Read the model definition and answer for the solid it produces. Units are mm, in the model's axes. Face numbers are marked on the shaded views. A direction names the side the tool comes from. Round coordinates to 2 decimals unless told otherwise and drop trailing zeros. Write each loop counter-clockwise with the first axis right and the second up, starting at its lowest first coordinate (ties: lowest second). Pieces come first, ordered by that corner, then holes.
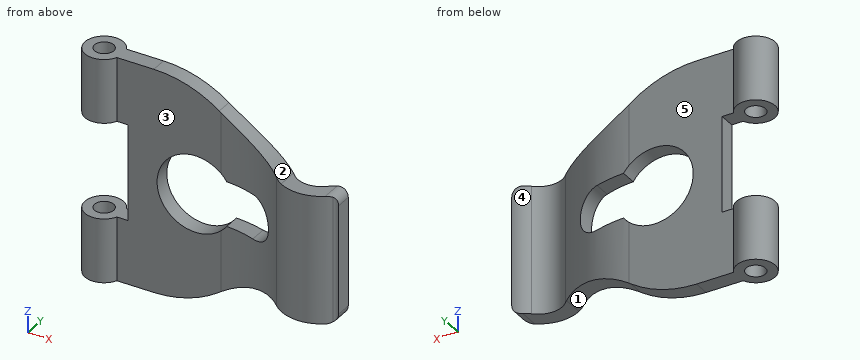
from build123d import *

# Parameters (mm, degrees)
SKETCH1_R               = 3
BOSS_EXTRUDE1_DEPTH     = 35
SKETCH2_W               = 15
SKETCH2_H               = 30
CUT_EXTRUDE2_DEPTH      = 4.5
CUT_EXTRUDE2_DEPTH_BACK = 19.180194847
CUT_EXTRUDE3_DEPTH      = 4.5
CUT_EXTRUDE3_DEPTH_BACK = 19.180194847
CUT_EXTRUDE5_DEPTH      = 4.5
CUT_EXTRUDE5_DEPTH_BACK = 19.180194847
FILLET2_R               = 3


with BuildPart() as part:
    # Sketch1 → Boss-Extrude1 (new body, symmetric)
    with BuildSketch(Plane.XY):
        with BuildLine():
            Line((6, -2.5), (38, -2.5))
            ThreePointArc((38, -2.5), (50.437211552, -4.973915193), (60.980970389, -12.019029611))
            ThreePointArc((60.980970389, -12.019029611), (69.818490023, -15.680194777), (78.656779847, -12.020889292))
            ThreePointArc((78.656779847, -12.020889292), (79.273086166, -11.609227247), (80, -11.464674847))
            Line((80, -11.464674847), (80, -6.464674847))
            ThreePointArc((80, -6.464674847), (77.360155024, -6.989628298), (75.121989969, -8.484611514))
            ThreePointArc((75.121989969, -8.484611514), (69.819016075, -10.680194805), (64.516504294, -8.483495706))
            ThreePointArc((64.516504294, -8.483495706), (52.350628714, -0.354517531), (38, 2.5))
            Line((38, 2.5), (6, 2.5))
            Line((6, 2.5), (5.454356057, 2.5))
            ThreePointArc((5.454356057, 2.5), (-6, 0), (5.454356057, -2.5))
            Line((5.454356057, -2.5), (6, -2.5))
        make_face()
        Circle(SKETCH1_R, mode=Mode.SUBTRACT)
    extrude(amount=BOSS_EXTRUDE1_DEPTH, both=True)

    # Sketch2 → Cut-Extrude2 (cut, two sides)
    with BuildSketch(Plane(origin=(0, 2.5, 0), x_dir=(1, 0, 0), z_dir=(0, 1, 0))) as cut_extrude2_sk:
        with Locations((1.5, 0)):
            Rectangle(SKETCH2_W, SKETCH2_H)
    extrude(amount=CUT_EXTRUDE2_DEPTH, mode=Mode.SUBTRACT)
    extrude(cut_extrude2_sk.sketch, amount=-CUT_EXTRUDE2_DEPTH_BACK, mode=Mode.SUBTRACT)

    # Sketch3 → Cut-Extrude3 (cut, two sides)
    with BuildSketch(Plane(origin=(0, 2.5, 0), x_dir=(1, 0, 0), z_dir=(0, 1, 0))) as cut_extrude3_sk:
        with BuildLine():
            Line((39.746794345, 7), (49, 7))
            ThreePointArc((49, 7), (56, 0), (49, -7))
            Line((49, -7), (39.746794345, -7))
            ThreePointArc((39.746794345, -7), (18, 0), (39.746794345, 7))
        make_face()
    extrude(amount=CUT_EXTRUDE3_DEPTH, mode=Mode.SUBTRACT)
    extrude(cut_extrude3_sk.sketch, amount=-CUT_EXTRUDE3_DEPTH_BACK, mode=Mode.SUBTRACT)

    # Sketch4 → Cut-Extrude5 (cut, two sides)
    with BuildSketch(Plane(origin=(0, 2.5, 0), x_dir=(1, 0, 0), z_dir=(0, 1, 0))) as cut_extrude5_sk:
        with BuildLine():
            Line((80, -20), (63.636895265, -20))
            ThreePointArc((63.636895265, -20), (49.858515462, -22.16127628), (37.403641679, -28.4375))
            ThreePointArc((37.403641679, -28.4375), (27.716517625, -33.319007338), (17, -35))
            Line((17, -35), (80, -35))
            Line((80, -35), (80, -20))
        make_face()
        with BuildLine():
            Line((80, 20), (63.636895265, 20))
            ThreePointArc((63.636895265, 20), (49.858515462, 22.16127628), (37.403641679, 28.4375))
            ThreePointArc((37.403641679, 28.4375), (27.716517625, 33.319007338), (17, 35))
            Line((17, 35), (80, 35))
            Line((80, 35), (80, 20))
        make_face()
    extrude(amount=CUT_EXTRUDE5_DEPTH, mode=Mode.SUBTRACT)
    extrude(cut_extrude5_sk.sketch, amount=-CUT_EXTRUDE5_DEPTH_BACK, mode=Mode.SUBTRACT)

    # Fillet2
    fillet2_edges = [part.edges().sort_by_distance(p)[0] for p in [
        (80, -8.964674847, -20),
        (80, -8.964674847, 20),
    ]]
    fillet(fillet2_edges, radius=FILLET2_R)


solid = part.part
Q1. Section B-B (z = 0) is taken. Determine the outline of the cut face in (x, y), then the cut area to 3 significant figures.
Verdict:
outline: (9, -2.5) - (18, -2.5) - (18, 2.5) - (9, 2.5) - close; (56, -7.94) arc R32.5 cw to (60.98, -12.02) arc R12.5 ccw to (78.66, -12.02) arc R1.9 cw to (80, -11.46) - (80, -6.46) arc R6.9 ccw to (75.12, -8.48) arc R7.5 cw to (64.52, -8.48) arc R37.5 ccw to (56, -2.1) - close
area: 184 mm2
Q2. Which of the six approach directions +Z, -Z, +X, -X, +Y, -Y give full straight-line access (tool end or side, diameter ignored) to the marked faces 1, 2, 3, 4 and 5?
Verdict:
face 1: -Z, +X, +Y, -Y
face 2: +Z, +X, +Y, -Y
face 3: +Z, -Z, -Y
face 4: +Z, -Z, +Y
face 5: +Z, -Z, +X, +Y
Q3. Straight lines are drawn through the part: probe 1 along Y at (x, z) = (0, -23); probe 2 along Z at (x, y) = (-1, 4.75); probe 3 along X at (y, z) = (0, 28.25). For each, find the intervals that lie inside material, in ascending order.
Verdict:
probe 1: y = -6 to -3, 3 to 6
probe 2: z = -35 to -15, 15 to 35
probe 3: x = -6 to -3, 3 to 37.67
Q4. Section C-C (x = 30) is taken. Determine the outline of the cut face in (y, z), then the cut area to 3 significant figures.
Verdict:
outline: (-2.5, -32.5) - (2.5, -32.5) - (2.5, -12) - (-2.5, -12) - close; (-2.5, 12) - (2.5, 12) - (2.5, 32.5) - (-2.5, 32.5) - close
area: 205 mm2
Q5. Section D-D (x = 45.5) is taken. Determine the outline of the cut face in (y, z).
Verdict:
outline: (-3.38, -23.82) - (1.74, -23.82) - (1.74, -7) - (-3.38, -7) - close; (-3.38, 7) - (1.74, 7) - (1.74, 23.82) - (-3.38, 23.82) - close
Q6. Section A-A (x = 0) is taken. Determine the outline of the cut face in (y, z).
Verdict:
outline: (-6, -35) - (-3, -35) - (-3, -15) - (-6, -15) - close; (-6, 15) - (-3, 15) - (-3, 35) - (-6, 35) - close; (3, -35) - (6, -35) - (6, -15) - (3, -15) - close; (3, 15) - (6, 15) - (6, 35) - (3, 35) - close
Q7. Flat-ended cylindrical pins translate along their axes: pin 1 Ø10 at (x, y) = (17, -3) entering from +Z; pin 2 Ø4.5 at (x, y) = (67.5, -12) entering from -Z; pin 3 Ø14.5 at (x, z) = (30, 0) entering from +Y; pin 4 Ø4 at (x, z) = (15.5, -13.5) entering from -Y. Find the tip coordinate at first contact, or state that the pin passes through.
Verdict:
pin 1: stops at z = 35
pin 2: stops at z = -20
pin 3: passes through
pin 4: stops at y = -2.5
